```python
from build123d import *

# Parameters (mm, degrees)
LENGTH_DEPTH       = 60
CUT_EXTRUDE1_DEPTH = 12


with BuildPart() as part:
    # Sketch1 → Length (new body)
    with BuildSketch(Plane(origin=(0, 0, 0), x_dir=(1, 0, 0), z_dir=(0, 1, 0))):
        with BuildLine():
            ThreePointArc((1.322875656, 1.5), (0, 2), (-1.322875656, 1.5))
            Line((-1.322875656, 1.5), (1.322875656, 1.5))
        make_face()
        with BuildLine():
            Line((1.322875656, 1.5), (-1.322875656, 1.5))
            ThreePointArc((-1.322875656, 1.5), (-0.822875656, -1.822875656), (2, 0))
            ThreePointArc((2, 0), (1.822875656, 0.822875656), (1.322875656, 1.5))
        make_face()
    extrude(amount=LENGTH_DEPTH)

    # Sketch1_3 → Cut-Extrude1 (cut)
    with BuildSketch(Plane(origin=(0, 0, 0), x_dir=(1, 0, 0), z_dir=(0, 1, 0))):
        Polygon((-20.975129822, 1.5), (-1.322875656, 1.5), (1.322875656, 1.5), (20.975129822, 1.5), (20.975129822, 40.804508332), (-20.975129822, 40.804508332), align=None)
    cut_extrude1 = extrude(amount=CUT_EXTRUDE1_DEPTH, mode=Mode.SUBTRACT)

    # Mirror1: Cut-Extrude1 across plane
    add(cut_extrude1.mirror(Plane(origin=(0, 30, 0), x_dir=(0, 0, 1), z_dir=(0, -1, 0))), mode=Mode.SUBTRACT)


solid = part.part
```
Source: CAD feature listing. Evaluate the final solid. Frame: model axes, mm. A direction names the side the tool comes from. Round coordinates to 2 decimals unless told otherwise and drop trailing zeros. Loops run counter-clockwise (first coordinate to the right, second up) from the corner with the lowest first, then second, coordinate; pieces in that order, holes last. Notation, with made-up numbers: M -5.5,17.5 L 21.5,17.5 A10 ccw 21.5,26.5 Z; hole C 69,-17 d1. An arc over 180 degrees is marked long. Use a Markdown table: item, result. Add a question column.
1. Section query D-D on y = 35. Return the cut outline in (x, z).
2. Section query C-C on z = 1.1. Return the cut outline in (x, y), then the cut area to 3 significant figures.
3. Section query A-A on x = 0.2. Return the cut outline in (y, z), then the cut area to 3 significant figures.
4. Contact query for flat-ended pins moving along their axis: P1, Ø1.3, axis at x = 0, y = 8.5, coming from the -Z side; P2, Ø1, axis at x = 1, y = 50, coming from the +Z side. Output: stop coordinate, or through.
5. Line query: line 1 (Z direction, x = -0.1, y = 55); line 2 (Z direction, x = -0.1, y = 15); line 3 (X direction, y = 23, z = 1.5). Output: solid intervals per line, ascending.
6. Reachability of faces 1 (the flat face through (0, 0, 0)), 2 (the flat face through (0, 6, -1.5)), 3 (the flat face through (0, 54, -1.5)) from +Z, -Z, +X, -X, +Y, -Y: full face, straight path, thin tool, end or side. Return the list, or none.
7. Section query B-B on y = 10. Return the cut outline in (x, z).
Reported:
| question | item | result |
|---|---|---|
| 1 | outline | C 0,0 d4 |
| 2 | outline | M -1.67,0 L 1.67,0 L 1.67,60 L -1.67,60 Z |
| 2 | area | 200 mm² |
| 3 | outline | M 0,-1.5 L 12,-1.5 L 12,-1.99 L 48,-1.99 L 48,-1.5 L 60,-1.5 L 60,1.99 L 0,1.99 Z |
| 3 | area | 227 mm² |
| 4 | P1 | stops at z = -1.5 |
| 4 | P2 | stops at z = 1.94 |
| 5 | line 1 | z = -1.5 to 2 |
| 5 | line 2 | z = -2 to 2 |
| 5 | line 3 | x = -1.32 to 1.32 |
| 6 | face 1 | +Z, -Z, +X, -X, -Y |
| 6 | face 2 | -Z, +X, -X, -Y |
| 6 | face 3 | -Z, +X, -X, +Y |
| 7 | outline | M -1.32,-1.5 L 1.32,-1.5 A2 ccw long Z |
